from build123d import *

# Parameters (mm, degrees)
F0_R     = 11
F0_R_2   = 6.75
F1_DEPTH = 40
F0_R_3   = 4
F2_DEPTH = 20
F3_SIZE2 = 19.99999
F3_SIZE  = 0.49999
F4_SIZE2 = 35
F4_SIZE  = 0.5


# Not quite as in the source:
# - a fillet or chamfer is up to 0.001 mm smaller than in the source, because OpenCascade refuses the exact size


with BuildPart() as f1:
    # F0 (on Top) → F1 (new body)
    with BuildSketch(Plane.XY):
        Circle(F0_R)
        Circle(F0_R_2, mode=Mode.SUBTRACT)
    extrude(amount=F1_DEPTH)

    # F0 (on Top) → F2 (join)
    with BuildSketch(Plane.XY):
        Circle(F0_R_2)
        Circle(F0_R_3, mode=Mode.SUBTRACT)
    extrude(amount=F2_DEPTH)

    # F3 (size 0.5 and 20 in the source; OpenCascade refuses exactly that, so slightly less here)
    f3_edges = [f1.edges().sort_by_distance(p)[0] for p in [
        (-6.75, 0, 40),
    ]]
    f3_side = f1.faces().sort_by_distance((-10.688873, 0, 40))[0]
    chamfer(f3_edges, length=F3_SIZE, length2=F3_SIZE2, reference=f3_side)

    # F4
    f4_edges = [f1.edges().sort_by_distance(p)[0] for p in [
        (-11, 0, 40),
    ]]
    f4_side = f1.faces().sort_by_distance((-7.561117, 0, 40))[0]
    chamfer(f4_edges, length=F4_SIZE, length2=F4_SIZE2, reference=f4_side)


solid = f1.part
Can you work these out from the model? Positions are in its coordinate system, mm. A direction names the side the tool comes from. Coordinates: 2 decimals unless noted, no trailing zeros. Write each loop counter-clockwise with the first axis right and the second up, starting at its lowest first coordinate (ties: lowest second). Pieces come first, ordered by that corner, then holes. Notation, with made-up numbers: (70, 72.5) - (127, 72.5) arc R5 cw to (127, 77.5) - close; hole circle Ø6 at (-18.75, 6). An arc over 180 degrees is marked (long way). Return JSON: item names as keys, results as strings. Group by question number.
Item 1: If we section it at A-A (z = 14): Write out the boundary of the cut face in (x, y).
Item 2: If we section it at B-B (z = 34.5): Write out the boundary of the cut face in (x, y), then the cut area to 3 significant figures.
Item 3: Please list where these lines run through material, in increasing order: probe 1 along Z at (x, y) = (4, -2.75); probe 2 along X at (y, z) = (5.25, 35); probe 3 along Y at (x, z) = (-3.75, 25.5).
Item 4: Which directions (+Z, -Z, +X, -X, +Y, -Y) give clear straight access to the entire face, cutting with the end or side of a thin tool? Please do faces 4 (the face through (0, -5, 0)), 5 (the face through (6.673, 2.102, 29.86)).
Item 5: I'm going to push flat-ended pins straight in: pin 1 Ø3 at (x, z) = (4, 33.5) entering from -Y; pin 2 Ø4 at (x, y) = (0, -1) entering from +Z; pin 3 Ø8 at (x, z) = (6.5, 14) entering from -Y; pin 4 Ø3 at (y, z) = (4.5, 32) entering from +X. Where does each tip first touch, or does it pass through?
Item 6: We'd pull the mould along Y, two halves only. Please class faces 1 (the face through (2.2, 7.1, 40)), 2 (the face through (-0.867, -3.905, 9.86)), 3 (the face through (-2.38, -10.74, 2.46)): pulls with the +Y half, pulls with the -Y half, needs draft (parallel to the pull), parting line crosses it, or undercut.
Return value:
{
 "1": {"outline": "circle Ø21.74 at (0, 0); hole circle Ø8 at (0, 0)"},
 "2": {"outline": "circle Ø21.16 at (0, 0); hole circle Ø14.22 at (0, 0)", "area": "193 mm^2"},
 "3": {"probe 1": "z = 0 to 20", "probe 2": "x = -9.18 to -4.82, 4.82 to 9.18", "probe 3": "y = -10.03 to -5.78, 5.78 to 10.03"},
 "4": {"face 4": "-Z, +X, -X, +Y, -Y", "face 5": "+Z"},
 "5": {"pin 1": "stops at y = -10.29", "pin 2": "passes through", "pin 3": "stops at y = -10.58", "pin 4": "stops at x = 10.18"},
 "6": {"face 1": "needs draft", "face 2": "undercut", "face 3": "parting line crosses it"}
}
